Source: CAD feature listing. Evaluate the final solid. Frame: model axes, mm. Face numbers are marked on the shaded views. Give positions to 0.01 mm unless a question says otherwise; leave off trailing zeros. Loops run counter-clockwise (first coordinate to the right, second up) from the corner with the lowest first, then second, coordinate; pieces in that order, holes last. Notation, with made-up numbers: (55, 37) - (60, 37) arc R28 cw to (60, 63) - close; hole circle Ø4 at (-39, 32.25). An arc over 180 degrees is marked (long way). Write each question's results on one line, items separated by ' | '. Start each with the question number.
(1) Cut plane B-B on y = 0. Return the cut outline in (x, z).
(2) Pull-direction query (X, two-part tool) for the marked faces 1, 2 and 3; classes: pulls with the +X half, pulls with the -X half, needs draft (parallel to the pull), parting line crosses it, or undercut.
(3) Material intervals for line 1 along Y through (x, z) = (0, -0.7); line 2 along Y through (x, z) = (0, 1.6), sorted ascending. Write a range as [from, to].
(4) Contact query for flat-ended pins moving along their axis: pin 1 (3.5 mm diameter, centred on x = 25, y = 0, fed in from +Z); pin 2 (4 mm diameter, centred on x = 10.5, y = -3, fed in from -Z); pin 3 (2.5 mm diameter, centred on x = 0, y = 0, fed in from -Z); pin 4 (1 mm diameter, centred on y = -1.5, z = 0, fed in from +X). Output: stop coordinate, or through.
(5) Cut plane A-A on x = 0. Return the cut outline in (y, z), then the cut area to 3 significant figures.
(6) Cut plane D-D on y = 3.25. Return the cut outline in (x, z), then the cut area to 3 significant figures.
(7) Cut plane C-C on z = -2.05. Return the cut outline in (x, y).
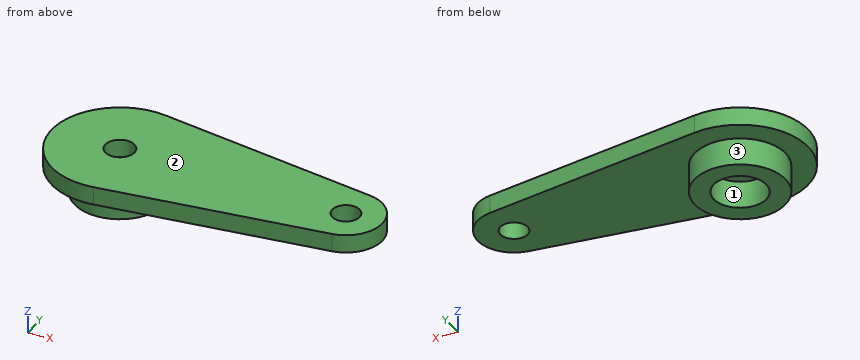
from build123d import *

# Parameters (mm, degrees)
F0_R     = 1.6
F0_R_2   = 1.5
F1_DEPTH = 2
F2_R     = 5
F2_R_2   = 2.9
F3_DEPTH = 3


with BuildPart() as f1:
    # F0 (on Top) → F1 (new body)
    with BuildSketch(Plane.XY):
        with BuildLine():
            Line((25.56, 3.960606), (1.05, 7.426136))
            ThreePointArc((1.05, 7.426136), (-7.5, 0), (1.05, -7.426136))
            Line((1.05, -7.426136), (25.56, -3.960606))
            ThreePointArc((25.56, -3.960606), (29, 0), (25.56, 3.960606))
        make_face()
        Circle(F0_R, mode=Mode.SUBTRACT)
        with Locations((25, 0)):
            Circle(F0_R_2, mode=Mode.SUBTRACT)
    extrude(amount=F1_DEPTH)

    # F2 (on face) → F3 (join)
    with BuildSketch(Plane(origin=(0, 0, 0), x_dir=(1, 0, 0), z_dir=(0, 0, -1))):
        Circle(F2_R)
        Circle(F2_R_2, mode=Mode.SUBTRACT)
    extrude(amount=F3_DEPTH)


solid = f1.part
Ans:
1) outline: (-7.5, 0) - (-5, 0) - (-5, -3) - (-2.9, -3) - (-2.9, 0) - (-1.6, 0) - (-1.6, 2) - (-7.5, 2) - close; (1.6, 0) - (2.9, 0) - (2.9, -3) - (5, -3) - (5, 0) - (23.5, 0) - (23.5, 2) - (1.6, 2) - close; (26.5, 0) - (29, 0) - (29, 2) - (26.5, 2) - close
2) face 1: undercut | face 2: needs draft | face 3: parting line crosses it
3) line 1: [-5, -2.9], [2.9, 5] | line 2: [-7.5, -1.6], [1.6, 7.5]
4) pin 1: z = 2 | pin 2: z = 0 | pin 3: through | pin 4: x = 28.87
5) outline: (-7.5, 0) - (-5, 0) - (-5, -3) - (-2.9, -3) - (-2.9, 0) - (-1.6, 0) - (-1.6, 2) - (-7.5, 2) - close; (1.6, 0) - (2.9, 0) - (2.9, -3) - (5, -3) - (5, 0) - (7.5, 0) - (7.5, 2) - (1.6, 2) - close | area: 36.2 mm^2
6) outline: (-6.76, 0) - (-3.8, 0) - (-3.8, -3) - (3.8, -3) - (3.8, 0) - (27.33, 0) - (27.33, 2) - (-6.76, 2) - close | area: 91.0 mm^2
7) outline: circle Ø10 at (0, 0); hole circle Ø5.8 at (0, 0)
